from build123d import *

# Parameters (mm, degrees)
F1_DEPTH = 5.85
F2_R     = 2
F3_R     = 0.365402
F4_W     = 6.1
F4_H     = 7.6
F5_DEPTH = 1.5


with BuildPart() as f1:
    # F0 (on Top) → F1 (new body, symmetric)
    with BuildSketch(Plane.XY):
        with BuildLine():
            Line((25, 1), (0, 1))
            Line((0, 1), (0, -1))
            Line((0, -1), (27, -1))
            Line((27, -1), (27, 3))
            Line((27, 3), (34, 1.765711))
            ThreePointArc((34, 1.765711), (35.583223, 3.829008), (34, 5.892305))
            Line((34, 5.892305), (28, 7.5))
            Line((28, 7.5), (27, 7.5))
            Line((27, 7.5), (27, 9))
            Line((27, 9), (25, 9))
            Line((25, 9), (25, 1))
        make_face()
    extrude(amount=F1_DEPTH, both=True)

    # F2
    f2_edges = [f1.edges().sort_by_distance(p)[0] for p in [
        (27, -1, 0),
    ]]
    fillet(f2_edges, radius=F2_R)

    # F3
    f3_edges = [f1.edges().sort_by_distance(p)[0] for p in [
        (27, 3, 0),
    ]]
    fillet(f3_edges, radius=F3_R)

    # F4 (on face) → F5 (cut)
    with BuildSketch(Plane(origin=(3.750644, 13.997595, 0), x_dir=(-0.965926, 0.258819, 0), z_dir=(0.258819, 0.965926, 0))):
        with Locations((-28.210609, 0)):
            Rectangle(F4_W, F4_H)
    extrude(amount=-F5_DEPTH, mode=Mode.SUBTRACT)


solid = f1.part
The model under review builds one solid part; all positions refer to its coordinate system, in mm. A direction names the side the tool comes from. Round coordinates to 2 decimals unless told otherwise and drop trailing zeros. Order: outer loops, then holes, each group sorted by start corner. A loop starts at its lowest first (then second) coordinate and runs counter-clockwise, first axis right, second up. Notation, with made-up numbers: (76, 14) -> (115, 14) arc R25 ccw to (115, 38) -> close; hole circle Ø2 at (-16.5, 10). An arc over 180 degrees is marked (long way). Write item = value, one per line. Start each with the question number.
Item 1: Mouldability with a two-part tool opening along X and no side actions: class faces 5 (the face through (30.668, 2.353, 0.082)), 6 (the face through (13, 1, 0)), 7 (the face through (27.863, 6.771, -0.053)) as released by +X, released by -X, zero draft, split by the parting line, or undercut.
Item 2: Consider section B-B on x = 29. Write out the cut boundary in (y, z), plus the area to 3 significant figures.
Item 3: For faces 1 (the face through (27, 8, 0)), 2 (the face through (33.755, 5.192, -0.053)), 3 (the face through (27, 2, 0)), 4 (the face through (25, 5, 0)), list the 3-axis set-ups (+Z, -Z, +X, -X, +Y, -Y) from which the entire face can be reached by the end or side of a thin tool; tool diameter is ignored.
Item 4: Clearance check with flat-ended pins moving along their axes: pin 1 Ø4 at (y, z) = (1.5, -3.5) entering from -X; pin 2 Ø1.2 at (y, z) = (8, -1) entering from +X; pin 3 Ø0.8 at (y, z) = (2, -2.5) entering from +X; pin 4 Ø0.5 at (x, z) = (27.5, -0.5) entering from +Y. State where each tip first meets the part, or that it passes through.
Item 5: Consider section C-C on y = 8.5. Write out the cut boundary in (x, z).
Item 6: Consider section A-A on z = -2.5. Write out the cut boundary in (x, y), plus the area to 3 significant figures.
Item 7: Consider section D-D on x = 4. Write out the cut boundary in (y, z), plus the area to 3 significant figures.
Item 8: For line 1 along X through (y, z) = (1.25, 4.25); line 2 along Y through (x, z) = (3.5, 2); line 3 along X through (y, z) = (4.25, 5), list the stretches that pass through material, from the lowest coordinate up.
Conclusion:
q1.face_5 = undercut
q1.face_6 = zero draft
q1.face_7 = released by +X
q2.outline = (2.65, -5.85) -> (7.23, -5.85) -> (7.23, -3.8) -> (5.68, -3.8) -> (5.68, 3.8) -> (7.23, 3.8) -> (7.23, 5.85) -> (2.65, 5.85) -> close
q2.area = 41.8 mm2
q3.face_1 = +Z, -Z, +X, +Y
q3.face_2 = +Y
q3.face_3 = +Z, -Z, -Y
q3.face_4 = +Z, -Z, -X, +Y
q4.pin_1 = 0
q4.pin_2 = 28.05
q4.pin_3 = 35.03
q4.pin_4 = 7.5
q5.outline = (25, -5.85) -> (27, -5.85) -> (27, 5.85) -> (25, 5.85) -> close
q6.outline = (0, -1) -> (25, -1) arc R2 ccw to (27, 1) -> (27, 2.56) arc R0.37 cw to (27.43, 2.92) -> (34, 1.77) arc R2.14 ccw to (34, 5.89) -> (33.95, 5.91) -> (33.56, 4.46) -> (27.67, 6.04) -> (28.05, 7.49) -> (28, 7.5) -> (27, 7.5) -> (27, 9) -> (25, 9) -> (25, 1) -> (0, 1) -> close
q6.area = 95.9 mm2
q7.outline = (-1, -5.85) -> (1, -5.85) -> (1, 5.85) -> (-1, 5.85) -> close
q7.area = 23.4 mm2
q8.line_1 = 25 to 27
q8.line_2 = -1 to 1
q8.line_3 = 25 to 35.54
